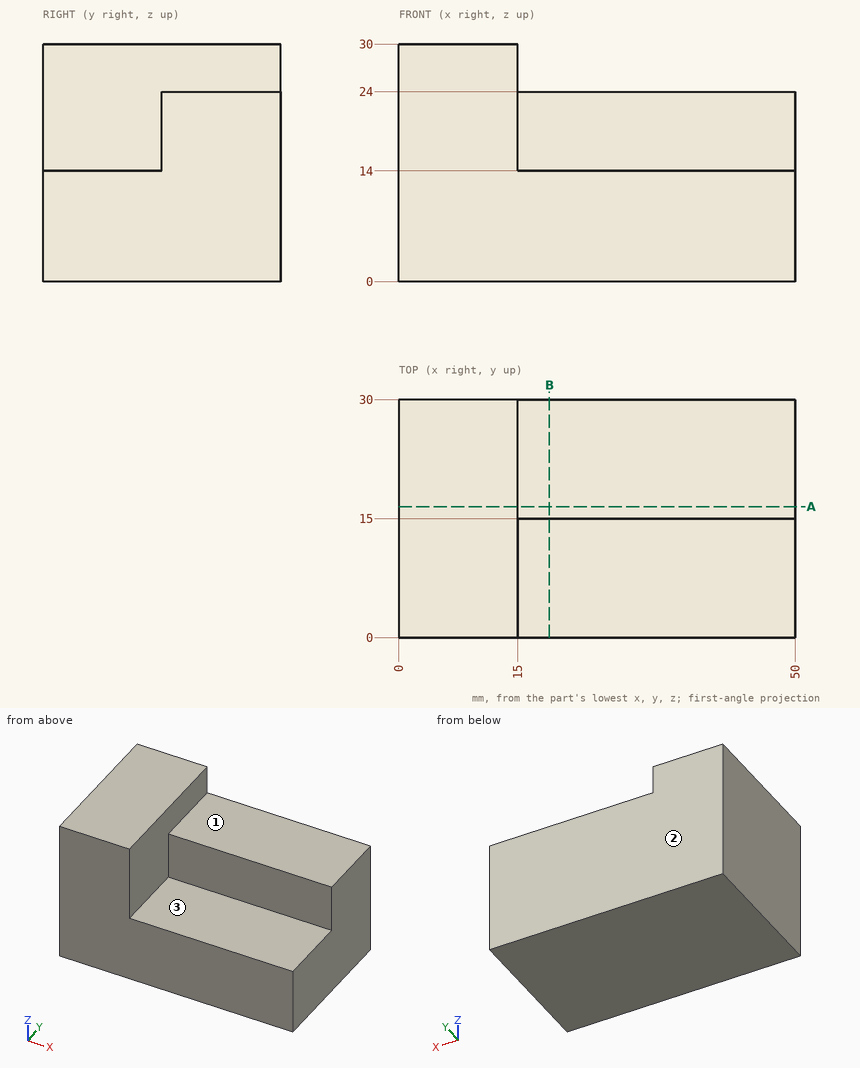
Can you work these out from the drawing? Everything is in mm from the part's minimum corner. A direction names the side the tool comes from. Round coordinates to 2 decimals unless told otherwise and drop trailing zeros. Loops run counter-clockwise (first coordinate to the right, second up) from the corner with the lowest first, then second, coordinate; pieces in that order, holes last. Notation, with made-up numbers: (2, -24.75) - (47, -24.75) arc R30 cw to (47, -1.75) - close; hole circle Ø3 at (34, 21.25). An arc over 180 degrees is marked (long way). One line per question, with ' | ' between items. Start each with the question number.
Q1. I want a section at B-B (x = 19). Write out the boundary of the cut face in (y, z), then the cut area to 3 significant figures.
Q2. For the marked faces 1, 2 and 3, which set-ups out of +Z, -Z, +X, -X, +Y, -Y let a thin tool reach every point of the face, with its end or its side?
Q3. I want a section at A-A (y = 16.5). Write out the boundary of the cut face in (x, z).
Q4. Will these pins go through, and if not, where does the flat tip stop? pin 1 (4.5 mm diameter, centred on x = 32, y = 22, fed in from +Z); pin 2 (8 mm diameter, centred on y = 9.5, z = 18.5, fed in from +X); pin 3 (6 mm diameter, centred on y = 25, z = 18.5, fed in from -X); pin 4 (11 mm diameter, centred on x = 35, z = 21.5, fed in from -Y).
Q5. Please list where these lines run through material, in increasing order: line 1 (Y direction, x = 42, z = 21.25); line 2 (Z direction, x = 39, y = 2.5); line 3 (X direction, y = 23, z = 28.5). Write a range as [from, to].
Response values:
1) outline: (0, 0) - (30, 0) - (30, 24) - (15, 24) - (15, 14) - (0, 14) - close | area: 570 mm²
2) face 1: +Z, +X, +Y, -Y | face 2: +Z, -Z, +X, -X, +Y | face 3: +Z, +X, -Y
3) outline: (0, 0) - (50, 0) - (50, 24) - (15, 24) - (15, 30) - (0, 30) - close
4) pin 1: stops at z = 24 | pin 2: stops at x = 15 | pin 3: stops at x = 0 | pin 4: stops at y = 15
5) line 1: y = [15, 30] | line 2: z = [0, 14] | line 3: x = [0, 15]
